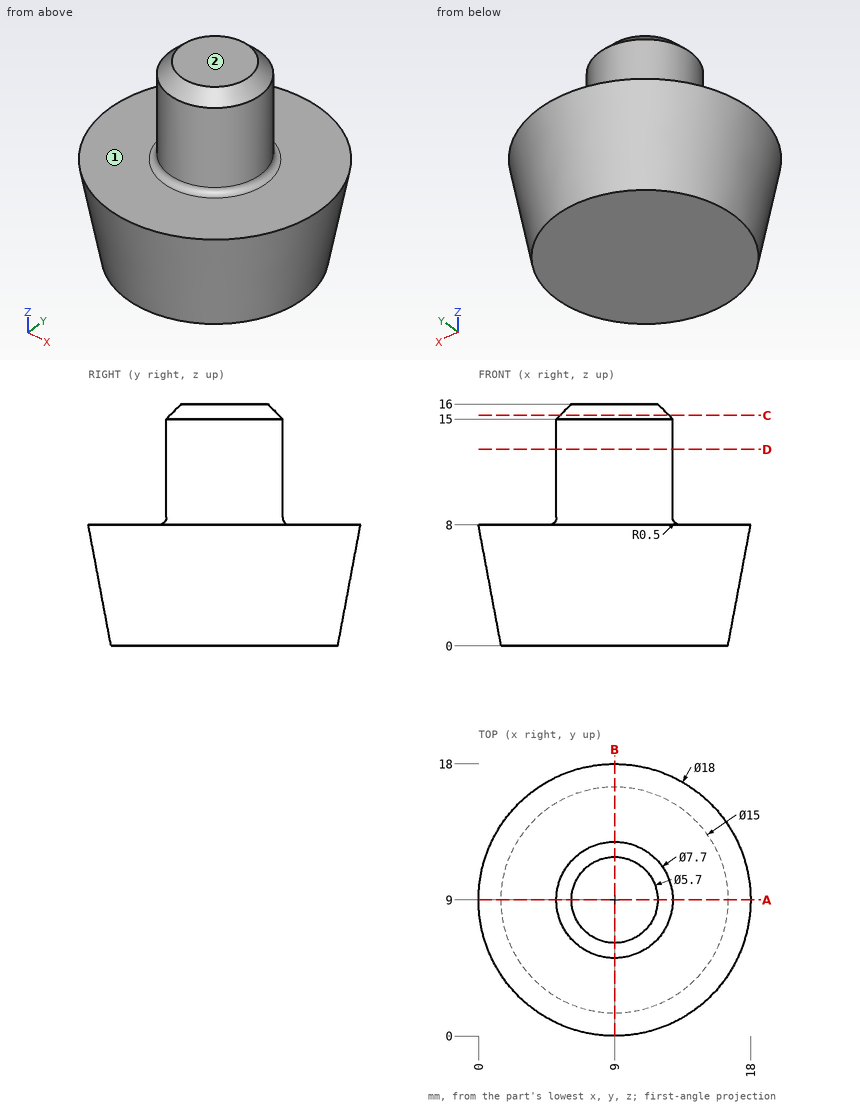
Could you check a few things on this drawing? It's one solid part, dimensions in mm from its lowest x, y, z. A direction names the side the tool comes from. Coordinates: 2 decimals unless noted, no trailing zeros. Write each loop counter-clockwise with the first axis right and the second up, starting at its lowest first coordinate (ties: lowest second). Pieces come first, ordered by that corner, then holes.
Q1. Which directions (+Z, -Z, +X, -X, +Y, -Y) give clear straight access to the entire face, cutting with the end or side of a thin tool? Please do the marked faces 1 and 2.
Results found:
face 1: +Z
face 2: +Z, +X, -X, +Y, -Y
Q2. Imagine slicing it at A-A, the plane y = 9. List the corners of the cut face in (x, z) for me, plus the area to 3 significant figures.
Results found:
outline: (0, 8) - (1.5, 0) - (16.5, 0) - (18, 8) - (13.35, 8) arc R0.5 cw to (12.85, 8.5) - (12.85, 15) - (11.85, 16) - (6.15, 16) - (5.15, 15) - (5.15, 8.5) arc R0.5 cw to (4.65, 8) - close
area: 193 mm2
Q3. Imagine slicing it at D-D, the plane z = 13. List the corners of the cut face in (x, y) for me.
Results found:
outline: circle Ø7.7 at (9, 9)
Q4. Imagine slicing it at C-C, the plane z = 15.25. List the corners of the cut face in (x, y) for me.
Results found:
outline: circle Ø7.2 at (9, 9)
Q5. Please list where these lines run through material, in increasing order: L1, parallel to Z at x = 3.5, y = 6; L2, parallel to X at y = 13.75, z = 6.5; L3, parallel to Y at x = 2.25, z = 1.5.
Results found:
L1: z = 0 to 8
L2: x = 1.69 to 16.31
L3: y = 5.13 to 12.87
Q6. For P1, Ø8, axis at y = 4.5, z = 14, coming from the +X side; P2, Ø6, axis at y = 14, z = 6.5, coming from the -X side; P3, Ø6, axis at x = 12.5, z = 13, coming from the -Y side, each with a flat end and sliding along its axis, tell me the tip position at first contact or that it passes through.
Results found:
P1: stops at x = 12.82
P2: stops at x = 0.33
P3: stops at y = 5.18
